Autodesk Inventor part; units mm, degrees
ref_plane "Work Plane1" through (0, 0, 13) normal (0, 0, 1) x (1, 0, 0)
ref_plane "YZ Plane" through (0, 0, 0) normal (1, 0, 0) x (0, 1, 0)
ref_plane "XZ Plane" through (0, 0, 0) normal (0, 1, 0) x (-1, 0, 0)
sketch "Sketch1" plane through (0, 0, 0) normal (0, 0, 1) x (1, 0, 0)
  line L0 (7.5517, 9.3259) -> (7.5517, -9.3259)
  line L1 (-7.5517, -9.3259) -> (-7.5517, 9.3259)
  line L2 (-7.5517, 9.3259) -> (7.5517, -9.3259) construction
  line L3 (7.5517, 9.3259) -> (-7.5517, -9.3259) construction
  arc A0 (-7.5517, -9.3259) -> (7.5517, -9.3259) centre (0, 0) ccw
  arc A1 (7.5517, 9.3259) -> (-7.5517, 9.3259) centre (0, 0) ccw
extrude "Extrusion1" add sketch "Sketch1" along normal blind 26
sketch "Sketch2" plane through (0, 0, 26) normal (0, 0, 1) x (1, 0, 0)
  circle A0 centre (0, 0) radius 7
  dimension "d3" = 14
extrude "Extrusion2" add sketch "Sketch2" along normal blind 3
sketch "Sketch3" plane through (0, 0, 29) normal (0, 0, 1) x (1, 0, 0)
  circle A0 centre (0, 0) radius 5
  dimension "d6" = 10
extrude "Extrusion3" add sketch "Sketch3" along normal blind 11.5
ref_plane "Work Plane1" through (0, 0, 13) normal (0, 0, 1) x (1, 0, 0)
mirror "Mirror1" about plane through (0, 0, 13) normal (0, 0, 1) of "Extrusion3", "Extrusion2"
sketch "Sketch4" plane through (-7.5517, -9.3259, 0) normal (-1, 0, 0) x (0, 0, 1)
  circle A0 centre (13, 9.3259) radius 6.5
  point P0 (0, 9.3259)
  dimension "d9" = 13
extrude "Extrusion4" cut sketch "Sketch4" against normal blind 100
thread "Thread1"
thread "Thread2"
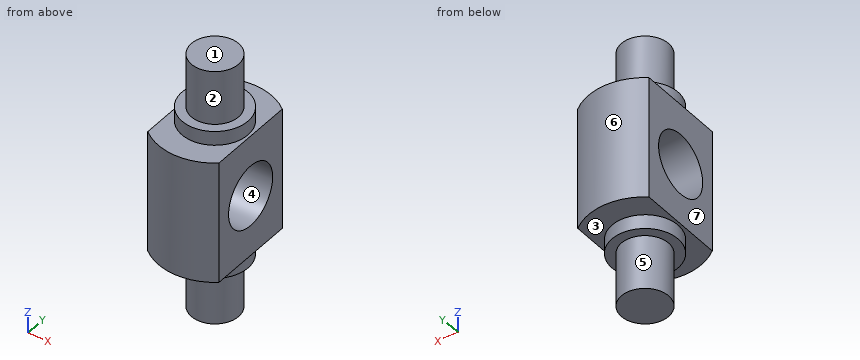
For this review, take the finished solid that the model builds, in its own axes (mm). Face numbers are marked on the shaded views. A direction names the side the tool comes from. Give positions to 0.01 mm unless a question says otherwise; leave off trailing zeros. Loops run counter-clockwise (first coordinate to the right, second up) from the corner with the lowest first, then second, coordinate; pieces in that order, holes last.
Item 1: Take a section at D-D, the plane z = 32.5. State the section outline as (x, y) points, and give its area (3 significant figures).
Item 2: Take a section at A-A, the plane y = 0. State the section outline as (x, z) points.
Item 3: Take a section at B-B, the plane z = 13. State the section outline as (x, y) points, and give its area (3 significant figures).
Item 4: Tool access review of the marked faces 1, 2 and 3: name each direction out of +Z, -Z, +X, -X, +Y, -Y from which nothing blocks a thin tool from reaching the whole face with its end or side.
Item 5: Take a section at C-C, the plane x = 0. State the section outline as (y, z) points, and give its area (3 significant figures).
Item 6: Insertion check: pin 1 (1.5 mm diameter, centred on x = -4, z = -4, fed in from -Y); pin 2 (6 mm diameter, centred on y = 7.5, z = 34.5, fed in from +X); pin 3 (4 mm diameter, centred on x = 3.5, z = 11, fed in from -Y). Each pin has a flat end and moves straight along its axis. Give the tip position at first contact, or say it passes through.
Item 7: For line 1 along Y through (x, z) = (-6.5, 19); line 2 along Z through (x, y) = (6.5, -1.25); line 3 along Z through (x, y) = (-6.5, 7.5), list the stretches that pass through material, from the lowest coordinate up.
Item 8: Draft analysis for pull direction Y (two halves, no side actions). For the marked faces 4, 5, 6 and 7, state which applies: +Y half, -Y half, draft (parallel to the pull), parting line (faces both ways), or undercut.
Calculated:
1. outline: circle Ø10 at (0, 0)
1. area: 78.5 mm2
2. outline: (-7.55, 0) - (-7, 0) - (-7, -3) - (-5, -3) - (-5, -14.5) - (5, -14.5) - (5, -3) - (7, -3) - (7, 0) - (7.55, 0) - (7.55, 6.5) - (-7.55, 6.5) - close; (-7.55, 19.5) - (7.55, 19.5) - (7.55, 26) - (7, 26) - (7, 29) - (5, 29) - (5, 40.5) - (-5, 40.5) - (-5, 29) - (-7, 29) - (-7, 26) - (-7.55, 26) - close
3. outline: (-7.55, -9.33) arc R12 ccw to (7.55, -9.33) - (7.55, -6.5) - (-7.55, -6.5) - close; (-7.55, 6.5) - (7.55, 6.5) - (7.55, 9.33) arc R12 ccw to (-7.55, 9.33) - close
3. area: 141 mm2
4. face 1: +Z, +X, -X, +Y, -Y
4. face 2: +Z
4. face 3: -Z
5. outline: (-12, 0) - (-7, 0) - (-7, -3) - (-5, -3) - (-5, -14.5) - (5, -14.5) - (5, -3) - (7, -3) - (7, 0) - (12, 0) - (12, 26) - (7, 26) - (7, 29) - (5, 29) - (5, 40.5) - (-5, 40.5) - (-5, 29) - (-7, 29) - (-7, 26) - (-12, 26) - close; hole circle Ø13 at (0, 13)
5. area: 805 mm2
6. pin 1: stops at y = -3.8
6. pin 2: stops at x = 2.18
6. pin 3: stops at y = -11.91
7. line 1: y = -10.09 to -2.5, 2.5 to 10.09
7. line 2: z = -3 to 6.62, 19.38 to 29
7. line 3: z = 0 to 26
8. face 4: undercut
8. face 5: parting line
8. face 6: +Y half
8. face 7: draft
